Solid Edge part; units mm, degrees
sketch "Sketch1" plane through (0, 0, 0) normal (0, -1, 0) x (1, 0, 0)
  line L0 (5, 2.8868) -> (0, 5.7735)
  line L1 (0, 5.7735) -> (-5, 2.8868)
  line L2 (-5, 2.8868) -> (-5, -2.8868)
  line L3 (-5, -2.8868) -> (0, -5.7735)
  line L4 (0, -5.7735) -> (5, -2.8868)
  line L5 (5, -2.8868) -> (5, 2.8868)
extrude "Protrusion1" add sketch "Sketch1" along normal mid plane 5.9
sketch "Sketch2" plane through (0, 0, 0) normal (1, 0, 0) x (0, 1, 0)
  line L0 (-2.95, 4.44) -> (-2.5927, 5.7735)
revolve "RevolvedCutout1" cut sketch "Sketch2" angle 360 about axis through (0, 0, 0) along (0, -1, 0) material side at (0, -2.8196, 5.1197)
hole "孔_7" at (0, -2.95, 0) direction (0, 1, 0) diameter 4.917 end up to next start chamfer 0.6 start chamfer angle 60 end chamfer 0.6 end chamfer angle 60
sketch "Sketch3" plane through (0, 0, 0) normal (1, 0, 0) x (0, 1, 0)
  line L0 (2.95, -4.6571) -> (1.0164, -5.7735)
revolve "RevolvedCutout2" cut sketch "Sketch3" angle 360 about axis through (0, 0, 0) along (0, 1, 0) material side at (0, 2.0082, -5.2586)
properties part number "N2531-"
CAD build for the part. Positions are in the model's coordinates, mm. Give positions to 0.01 mm unless a question says otherwise; leave off trailing zeros. Write each loop counter-clockwise with the first axis right and the second up, starting at its lowest first coordinate (ties: lowest second). Pieces come first, ordered by that corner, then holes. Notation, with made-up numbers: (3, 87) -> (20, 87) arc R27 cw to (20, 116) -> close; hole circle Ø2 at (80.5, -25). An arc over 180 degrees is marked (long way). Return JSON: item names as keys, results as strings.
Item 1: Two-plate mould, pull along Z, no slides. Class faces 1 (the flat face through (-2.535, -0.186, -4.31)), 2 (the cylindrical face through (0.738, -0.036, -2.345)), 3 (the flat face through (5, 0, 0)): +Z half, -Z half, draft (parallel to the pull), parting line (faces both ways), or undercut.
Answer below:
{"face 1": "-Z half", "face 2": "undercut", "face 3": "draft"}
Item 2: Band-saw the part on B-B (y = -2.45). List the corners of the cut face in (x, z), then the cut area to 3 significant figures.
Answer below:
{"outline": "(-5, -2.89) -> (0, -5.77) -> (5, -2.89) -> (5, 2.89) -> (0, 5.77) -> (-5, 2.89) -> close; hole circle Ø4.92 at (0, 0)", "area": "67.6 mm2"}
Item 3: Drop flat-ended pins along their axis: pin 1 (3 mm diameter, centred on x = 0, z = 0, fed in from +Y); pin 2 (1.5 mm diameter, centred on y = -1.5, z = 3, fed in from +X); pin 3 (1 mm diameter, centred on y = 2.5, z = -4.5, fed in from -X). Give the stop position or say it passes through.
Answer below:
{"pin 1": "passes through", "pin 2": "stops at x = 5", "pin 3": "stops at x = -3"}
Item 4: Band-saw the part on C-C (y = 2). List the corners of the cut face in (x, z).
Answer below:
{"outline": "(-5, -1.45) arc R5.21 ccw to (-3.75, -3.61) -> (-1.25, -5.05) arc R5.21 ccw to (1.25, -5.05) -> (3.75, -3.61) arc R5.21 ccw to (5, -1.45) -> (5, 1.45) arc R5.21 ccw to (3.75, 3.61) -> (1.25, 5.05) arc R5.21 ccw to (-1.25, 5.05) -> (-3.75, 3.61) arc R5.21 ccw to (-5, 1.45) -> close; hole circle Ø4.92 at (0, 0)"}
Item 5: Drill centre lines: probe 1 along X at (y, z) = (1.2, 0); probe 2 along X at (y, z) = (2.5, -0.25); probe 3 along Z at (x, y) = (1.5, -0.2). Where is each one in solid material? Low to high.
Answer below:
{"probe 1": "x = -5 to -2.46, 2.46 to 5", "probe 2": "x = -4.91 to -2.45, 2.45 to 4.91", "probe 3": "z = -4.91 to -1.95, 1.95 to 4.91"}
Item 6: Band-saw the part on A-A (z = 0). List the corners of the cut face in (x, y).
Answer below:
{"outline": "(-5, -2.8) -> (-4.44, -2.95) -> (-3.06, -2.95) -> (-2.46, -2.6) -> (-2.46, 2.6) -> (-3.06, 2.95) -> (-4.66, 2.95) -> (-5, 2.36) -> close; (2.46, -2.6) -> (3.06, -2.95) -> (4.44, -2.95) -> (5, -2.8) -> (5, 2.36) -> (4.66, 2.95) -> (3.06, 2.95) -> (2.46, 2.6) -> close"}
